from build123d import *

# Parameters (mm, degrees)
SKETCH_1_R          = 18.5
EXTRUDE_1_DEPTH     = 22
SKETCH_2_R          = 20
EXTRUDE_2_DEPTH     = 22
SKETCH_3_R          = 1.5
CUT_EXTRUDE_1_DEPTH = 5
SKETCH_4_R          = 4
EXTRUDE_3_DEPTH     = 6
EXTRUDE_4_DEPTH     = 12


with BuildPart() as part:
    # 草图1 → 凸台-拉伸1 (new body)
    with BuildSketch(Plane(origin=(0, 0, 0), x_dir=(1, 0, 0), z_dir=(0, 1, 0))):
        with Locations(Location((0, 0, 0), (0, 0, 270))):
            Circle(SKETCH_1_R)
    extrude(amount=EXTRUDE_1_DEPTH)

    # 草图2 → 凸台-拉伸2 (add)
    with BuildSketch(Plane(origin=(0, 22, 0), x_dir=(1, 0, 0), z_dir=(0, 1, 0))):
        with Locations(Location((0, 0, 0), (0, 0, 270))):
            Circle(SKETCH_2_R)
    extrude(amount=EXTRUDE_2_DEPTH)

    # 草图3 → 切除-拉伸1 (cut)
    with BuildSketch(Plane(origin=(0, 44, 0), x_dir=(1, 0, 0), z_dir=(0, 1, 0))):
        with Locations(Location((-7.75, 13.423393759, 0), (0, 0, 270))):
            Circle(SKETCH_3_R)
        with Locations(Location((-15.5, 0, 0), (0, 0, 270))):
            Circle(SKETCH_3_R)
        with Locations(Location((-7.75, -13.423393759, 0), (0, 0, 270))):
            Circle(SKETCH_3_R)
        with Locations(Location((7.75, -13.423393759, 0), (0, 0, 270))):
            Circle(SKETCH_3_R)
        with Locations(Location((15.5, 0, 0), (0, 0, 270))):
            Circle(SKETCH_3_R)
        with Locations(Location((7.75, 13.423393759, 0), (0, 0, 270))):
            Circle(SKETCH_3_R)
    extrude(amount=-CUT_EXTRUDE_1_DEPTH, mode=Mode.SUBTRACT)

    # 草图4 → 凸台-拉伸3 (add)
    with BuildSketch(Plane(origin=(0, 44, 0), x_dir=(1, 0, 0), z_dir=(0, 1, 0))):
        with Locations(Location((0, 7, 0), (0, 0, 270))):
            Circle(SKETCH_4_R)
    extrude(amount=EXTRUDE_3_DEPTH)

    # 草图5 → 凸台-拉伸4 (add)
    with BuildSketch(Plane(origin=(0, 50, 0), x_dir=(1, 0, 0), z_dir=(0, 1, 0))):
        with BuildLine():
            Line((2.4, 8.8), (2.4, 5.2))
            ThreePointArc((2.4, 5.2), (-3, 7), (2.4, 8.8))
        make_face()
    extrude(amount=EXTRUDE_4_DEPTH)


solid = part.part
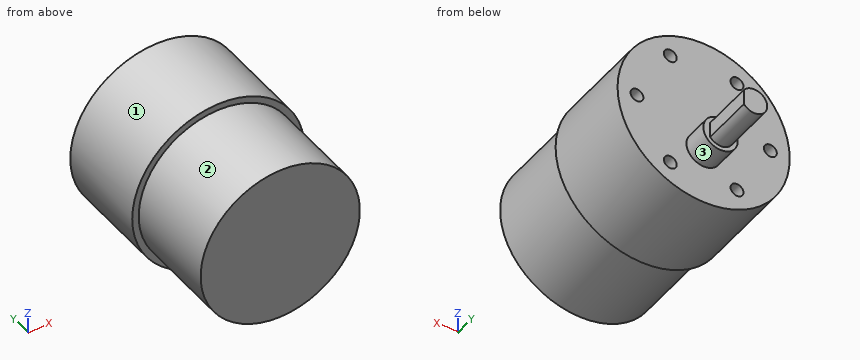
Verification items for the finished model (mm, model axes). Face numbers are marked on the shaded views. A direction names the side the tool comes from. Give positions to 0.01 mm unless a question says otherwise; leave off trailing zeros. Order: outer loops, then holes, each group sorted by start corner. A loop starts at its lowest first (then second) coordinate and runs counter-clockwise, first axis right, second up. Notation, with made-up numbers: M -1,45 L 42,45 A34 ccw 42,82 Z; hole C 72.25,83.25 d2. An arc over 180 degrees is marked long. Answer as a JSON object with one key per item and string values. Group by question number.
1) Access from +Z, -Z, +X, -X, +Y, -Y to the whole of each face (thin tool, end or side, straight path). Record for the marked faces 1, 2 and 3.
2) Depth check by flat-ended pin: pin 1 Ø1.5 at (x, z) = (8.5, -12.5) entering from +Y; pin 2 Ø8 at (y, z) = (14, -6) entering from +X; pin 3 Ø1.5 at (x, z) = (15.5, 0) entering from +Y; pin 4 Ø12 at (x, z) = (2, -10.5) entering from -Y. Enter the tip coordinate at first touch or a pass-through.
3) Cross-section at D-D (z = 5.5). Enter the section's corners in (x, y).
4) Cross-section at B-B (z = -7). Enter the section's corners in (x, y) (3 decimals), then the cut area to 3 significant figures.
5) Cross-section at C-C (y = 5). Enter the section's corners in (x, z).
6) Scan lines: line 1 along X through (y, z) = (39.5, 0); line 2 along Z through (x, y) = (-7, 40) (3 decimals); line 3 along Y through (x, z) = (10, -10.5). Record each from-to range of solid material in increasing order. Write a range as [from, to].
7) Cross-section at A-A (x = 0). Enter the section's corners in (y, z), then the cut area to 3 significant figures.
Result sheet:
{
 "1": {"face 1": "+Y, -Y", "face 2": "-Y", "face 3": "+Y"},
 "2": {"pin 1": "stops at y = 44", "pin 2": "stops at x = 18.39", "pin 3": "stops at y = 39", "pin 4": "stops at y = 0"},
 "3": {"outline": "M -19.23,22 L -17.66,22 L -17.66,0 L 17.66,0 L 17.66,22 L 19.23,22 L 19.23,44 L -19.23,44 Z"},
 "4": {"outline": "M -18.735,22 L -17.125,22 L -17.125,0 L 17.125,0 L 17.125,22 L 18.735,22 L 18.735,44 L 4,44 L 4,50 L 2.4,50 L 2.4,62 L -3,62 L -3,50 L -4,50 L -4,44 L -18.735,44 Z", "area": "1,690 mm2"},
 "5": {"outline": "C 0,0 d37"},
 "6": {"line 1": "x = [-20, -17], [-14, 14], [17, 20]", "line 2": "z = [-18.735, -14.722], [-12.124, 12.124], [14.722, 18.735]", "line 3": "y = [0, 44]"},
 "7": {"outline": "M 0,-18.5 L 22,-18.5 L 22,-20 L 44,-20 L 44,-11 L 50,-11 L 50,-10 L 62,-10 L 62,-4 L 50,-4 L 50,-3 L 44,-3 L 44,20 L 22,20 L 22,18.5 L 0,18.5 Z", "area": "1,810 mm2"}
}
